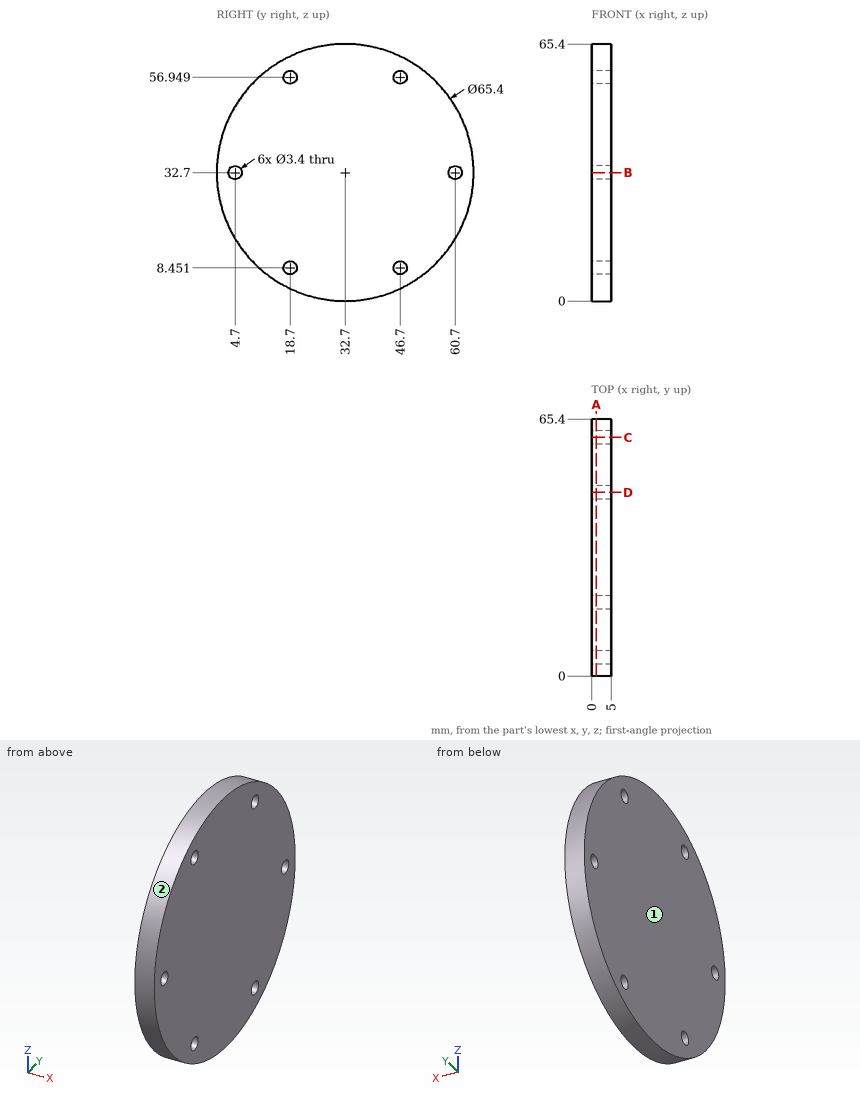
Geometry: see drawing. Coordinates: mm, zero at the bounding-box minimum. Give positions to 0.01 mm unless a question says otherwise; leave off trailing zeros. Order: outer loops, then holes, each group sorted by start corner. A loop starts at its lowest first (then second) coordinate and runs counter-clockwise, first axis right, second up. Notation, with made-up numbers: (82, -12.75) - (102, -12.75) arc R12 ccw to (102, 6.25) - close; hole circle Ø9 at (41, 12.25). An arc over 180 degrees is marked (long way). Write each question's results on one line, items separated by ' | '.
Item 1: Section B-B (z = 32.7). Return loops of the section in (x, y).
A:
outline: (0, 0) - (5, 0) - (5, 3) - (0, 3) - close; (0, 6.4) - (5, 6.4) - (5, 59) - (0, 59) - close; (0, 62.4) - (5, 62.4) - (5, 65.4) - (0, 65.4) - close
Item 2: Section D-D (y = 46.7). Return loops of the section in (x, z).
A:
outline: (0, 3.15) - (5, 3.15) - (5, 6.75) - (0, 6.75) - close; (0, 10.15) - (5, 10.15) - (5, 55.25) - (0, 55.25) - close; (0, 58.65) - (5, 58.65) - (5, 62.25) - (0, 62.25) - close
Item 3: Draft query along Y for the marked faces 1 and 2. Return one class per face: released by +Y, released by -Y, zero draft, split by the parting line, or undercut.
A:
face 1: zero draft | face 2: split by the parting line
Item 4: Contact query for flat-ended pins moving along their axis: pin 1 Ø2 at (x, z) = (2.5, 47) entering from -Y; pin 2 Ø3 at (x, z) = (1, 24.5) entering from +Y. Output: stop coordinate, or through.
A:
pin 1: stops at y = 2.83 | pin 2: stops at y = 64.71
Item 5: Material intervals for line 1 along Y through (x, z) = (3.25, 32.7); line 2 along Y through (x, z) = (2.4, 34) (1 decimal); line 3 along Z through (x, y) = (0.35, 33.5), sorted ascending.
A:
line 1: y = 0 to 3, 6.4 to 59, 62.4 to 65.4 | line 2: y = 0 to 3.6, 5.8 to 59.6, 61.8 to 65.4 | line 3: z = 0.01 to 65.39
Item 6: Section C-C (y = 60.7). Return loops of the section in (x, z), and give its area (3 significant figures).
A:
outline: (0, 15.81) - (5, 15.81) - (5, 31) - (0, 31) - close; (0, 34.4) - (5, 34.4) - (5, 49.59) - (0, 49.59) - close | area: 152 mm^2
Item 7: Section A-A (x = 1.2). Return loops of the section in (y, z).
A:
outline: circle Ø65.4 at (32.7, 32.7); hole circle Ø3.4 at (4.7, 32.7); hole circle Ø3.4 at (18.7, 8.45); hole circle Ø3.4 at (18.7, 56.95); hole circle Ø3.4 at (46.7, 8.45); hole circle Ø3.4 at (46.7, 56.95); hole circle Ø3.4 at (60.7, 32.7)
